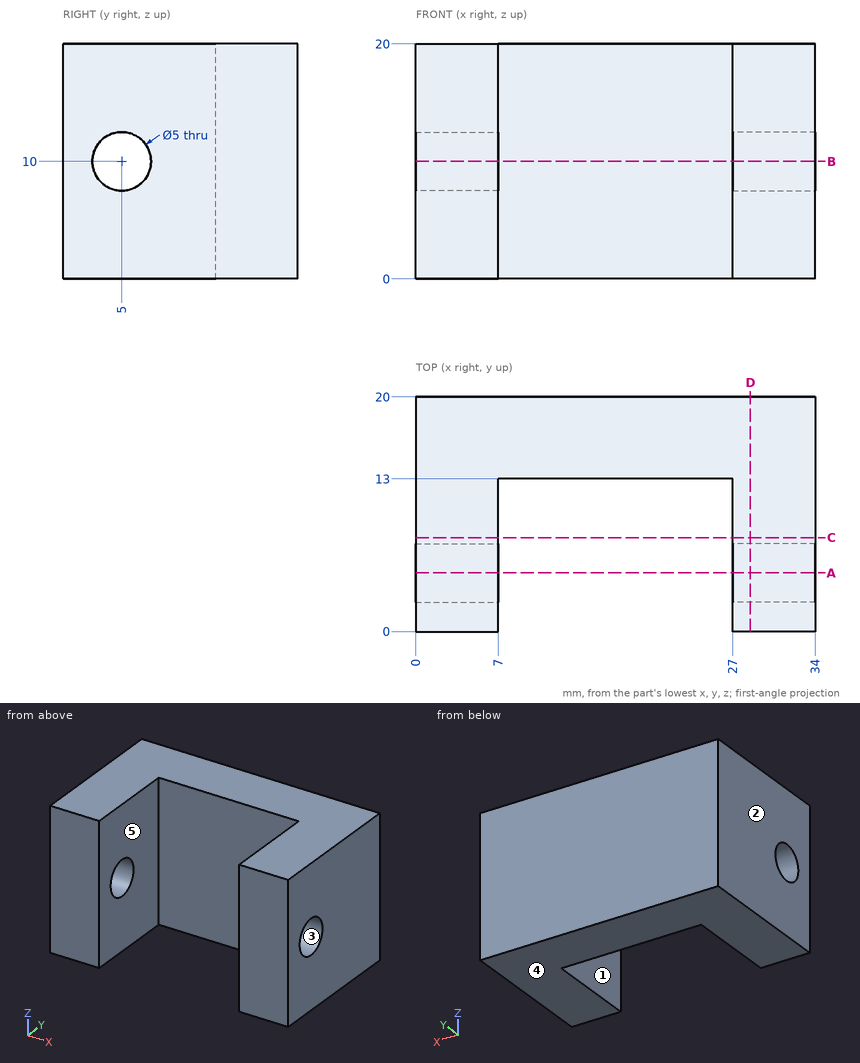
Here's the drawing with two shaded views (mm, measured from the low corner). I have some questions. A direction names the side the tool comes from. Coordinates: 2 decimals unless noted, no trailing zeros. Loops run counter-clockwise (first coordinate to the right, second up) from the corner with the lowest first, then second, coordinate; pieces in that order, holes last. Notation, with made-up numbers: M 9.5,79 L 32.5,79 A28 ccw 32.5,108 Z; hole C 33,39.25 d2. An arc over 180 degrees is marked long. Return JSON: item names as keys, results as strings. Group by question number.
Item 1: On a 3-axis mill with a long thin cutter (end or side, diameter ignored), from which of +Z, -Z, +X, -X, +Y, -Y can I reach the whole of each face in a straight line? I mean the marked faces 1 and 2. Say none if no direction works.
Item 2: Imagine slicing it at A-A (y = 5). Please give me the cut outline in (x, z), and give its area (3 significant figures).
Item 3: If I drill on L1, parallel to X at y = 11.75, z = 10; L2, parallel to Z at x = 32, y = 5; L3, parallel to Y at x = 30, z = 10, over which ranges is the centre line in solid material (lowest first)? Write a range as from..to.
Item 4: I'm going to push flat-ended pins straight in: pin 1 Ø6 at (y, z) = (5, 10) entering from -X; pin 2 Ø5 at (x, z) = (15, 11.5) entering from -Y. Where does each tip first touch, or does it pass through?
Item 5: Thinking about a two-plate mould opening in Z: for the marked faces 3, 4 and 5, which applies, released by +Z, released by -Z, zero draft, split by the parting line, or undercut?
Item 6: Imagine slicing it at B-B (z = 10). Please give me the cut outline in (x, y).
Item 7: Imagine slicing it at C-C (y = 8). Please give me the cut outline in (x, z).
Item 8: Imagine slicing it at D-D (x = 28.5). Please give me the cut outline in (y, z).
Verdict:
{
 "1": {"face 1": "+Z, -Z, -Y", "face 2": "+Z, -Z, -X, +Y, -Y"},
 "2": {"outline": "M 0,0 L 7,0 L 7,7.5 L 0,7.5 Z; M 0,12.5 L 7,12.5 L 7,20 L 0,20 Z; M 27,0 L 34,0 L 34,7.5 L 27,7.5 Z; M 27,12.5 L 34,12.5 L 34,20 L 27,20 Z", "area": "210 mm^2"},
 "3": {"L1": "x = 0..7, 27..34", "L2": "z = 0..7.5, 12.5..20", "L3": "y = 0..2.5, 7.5..20"},
 "4": {"pin 1": "stops at x = 0", "pin 2": "stops at y = 13"},
 "5": {"face 3": "undercut", "face 4": "released by -Z", "face 5": "zero draft"},
 "6": {"outline": "M 0,0 L 7,0 L 7,2.5 L 0,2.5 Z; M 0,7.5 L 7,7.5 L 7,13 L 27,13 L 27,7.5 L 34,7.5 L 34,20 L 0,20 Z; M 27,0 L 34,0 L 34,2.5 L 27,2.5 Z"},
 "7": {"outline": "M 0,0 L 7,0 L 7,20 L 0,20 Z; M 27,0 L 34,0 L 34,20 L 27,20 Z"},
 "8": {"outline": "M 0,0 L 20,0 L 20,20 L 0,20 Z; hole C 5,10 d5"}
}
